Design review of the part shown in the three views and the two pictorial views. Dimensions are in mm from the part's minimum x, y and z. A direction names the side the tool comes from. Give positions to 0.01 mm unless a question says otherwise; leave off trailing zeros. Write each loop counter-clockwise with the first axis right and the second up, starting at its lowest first coordinate (ties: lowest second). Pieces come first, ordered by that corner, then holes.
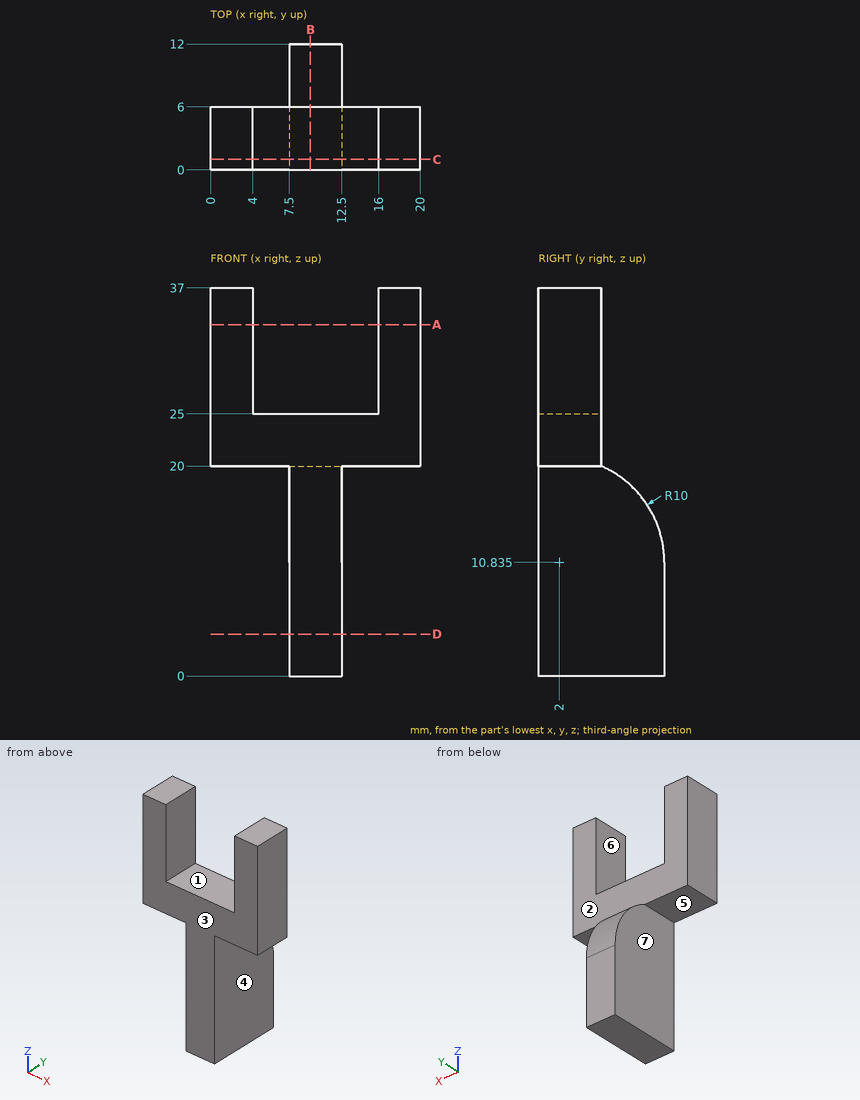
(1) To check wall thickness, follow L1, parallel to X at y = 2, z = 28; L2, parallel to X at y = 9.25, z = 9; L3, parallel to Z at x = 5.25, y = 3. State the ranges of each line that lie inside material, in increasing order.
Resolved:
L1: x = 0 to 4, 16 to 20
L2: x = 7.5 to 12.5
L3: z = 20 to 25
(2) Consider section A-A, the plane z = 33.5. Give the boundary of the cut face in (x, y), then the cut area to 3 significant figures.
Resolved:
outline: (0, 0) - (4, 0) - (4, 6) - (0, 6) - close; (16, 0) - (20, 0) - (20, 6) - (16, 6) - close
area: 48.0 mm2
(3) Consider section B-B, the plane x = 9.5. Give the boundary of the cut face in (y, z) (3 decimals), then the cut area to 3 significant figures.
Resolved:
outline: (0, 0) - (12, 0) - (12, 10.835) arc R10 ccw to (6, 20) - (6, 25) - (0, 25) - close
area: 255 mm2
(4) Consider section D-D, the plane z = 4. Give the boundary of the cut face in (x, y), then the cut area to 3 significant figures.
Resolved:
outline: (7.5, 0) - (12.5, 0) - (12.5, 12) - (7.5, 12) - close
area: 60.0 mm2
(5) Mouldability with a two-part tool opening along X and no side actions: class the marked faces 5, 6 and 7 as pulls with the +X half, pulls with the -X half, needs draft (parallel to the pull), parting line crosses it, or undercut.
Resolved:
face 5: needs draft
face 6: undercut
face 7: pulls with the -X half
(6) Consider section C-C, the plane y = 1. Give the boundary of the cut face in (x, z).
Resolved:
outline: (0, 20) - (7.5, 20) - (7.5, 0) - (12.5, 0) - (12.5, 20) - (20, 20) - (20, 37) - (16, 37) - (16, 25) - (4, 25) - (4, 37) - (0, 37) - close
(7) Clearance check with flat-ended pins moving along their axes: P1, Ø6.5, axis at x = 2.5, y = 4.5, coming from the -Z side; P2, Ø8.5, axis at x = 11.5, z = 29, coming from the +Y side; P3, Ø1, axis at y = 7, z = 6.5, coming from the -X side. State where each tip first meets the part, or that it passes through.
Resolved:
P1: stops at z = 20
P2: stops at y = 6
P3: stops at x = 7.5
(8) Tool access review of the marked faces 1, 2, 3 and 4: name each direction out of +Z, -Z, +X, -X, +Y, -Y from which nothing blocks a thin tool from reaching the whole face with its end or side.
Resolved:
face 1: +Z, +Y, -Y
face 2: +Z, +X, -X, +Y
face 3: +Z, -Z, +X, -X, -Y
face 4: -Z, +X, +Y, -Y
